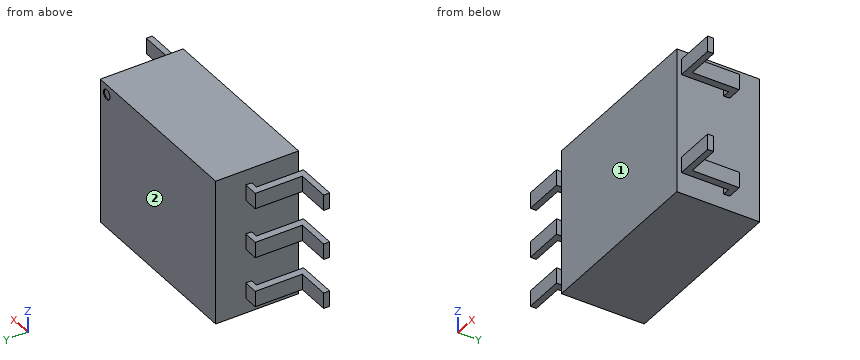
Autodesk Inventor part; units mm, degrees
ref_plane "YZ Plane" through (0, 0, 0) normal (1, 0, 0) x (0, 1, 0)
ref_plane "XZ Plane" through (0, 0, 0) normal (0, 1, 0) x (-1, 0, 0)
ref_plane "XY Plane" through (0, 0, 0) normal (0, 0, 1) x (1, 0, 0)
sketch "Sketch1" plane through (0, 0, 0) normal (0, 0, 1) x (1, 0, 0)
  line L0 (0, 0) -> (4.5491, 0)
  line L1 (4.5491, 0) -> (4.5491, 2.1006)
  line L2 (4.5491, 2.1006) -> (0, 2.1006)
  line L3 (0, 2.1006) -> (0, 0)
  dimension "d0" = 2.1006
  dimension "d1" = 4.5491
extrude "Extrusion1" add sketch "Sketch1" along normal blind 3.7008
sketch "Sketch2" plane through (4.5491, 0, 0) normal (1, 0, 0) x (0, 0, -1)
  line L0 (-3.3198, 1.3386) -> (-2.921, 1.3386)
  line L1 (-2.921, 1.3386) -> (-2.921, 1.1887)
  line L2 (-2.921, 1.1887) -> (-3.3198, 1.1887)
  line L3 (-3.3198, 1.1887) -> (-3.3198, 1.3386)
  line L4 (-0.7798, 1.3386) -> (-0.381, 1.3386)
  line L5 (-0.381, 1.3386) -> (-0.381, 1.1887)
  line L6 (-0.381, 1.1887) -> (-0.7798, 1.1887)
  line L7 (-0.7798, 1.1887) -> (-0.7798, 1.3386)
  line L8 (0, 0) -> (0, 2.1006)
  line L9 (0, 2.1006) -> (-3.7008, 2.1006)
  dimension "d4" = 0.3988
  dimension "d5" = 0.3988
  dimension "d6" = 0.1499
  dimension "d7" = 0.1499
  dimension "d8" = 2.1412
  dimension "d9" = 0
  dimension "d10" = 0.381
  dimension "d11" = 0.762
extrude "Extrusion2" add sketch "Sketch2" against normal blind 4.7727
extrude "Extrusion3" add sketch "Sketch2" along normal blind 0.2286
sketch "Sketch3" plane through (4.7777, 0, 0) normal (1, 0, 0) x (0, 0, -1)
  line L0 (-3.3198, 1.3386) -> (-2.921, 1.3386)
  line L1 (-2.921, 1.3386) -> (-2.921, 1.1887)
  line L2 (-2.921, 1.1887) -> (-3.3198, 1.1887)
  line L3 (-3.3198, 1.1887) -> (-3.3198, 1.3386)
  line L4 (-0.7798, 1.3386) -> (-0.381, 1.3386)
  line L5 (-0.381, 1.3386) -> (-0.381, 1.1887)
  line L6 (-0.381, 1.1887) -> (-0.7798, 1.1887)
  line L7 (-0.7798, 1.1887) -> (-0.7798, 1.3386)
  point P0 (0, 0)
extrude "Extrusion4" add sketch "Sketch3" along normal blind 0.1524
sketch "Sketch4" plane through (-0.2235, 0, 0) normal (-1, 0, 0) x (0, 0, 1)
  line L0 (2.921, 1.3386) -> (3.3198, 1.3386)
  line L1 (3.3198, 1.3386) -> (3.3198, 1.1887)
  line L2 (3.3198, 1.1887) -> (2.921, 1.1887)
  line L3 (2.921, 1.1887) -> (2.921, 1.3386)
  line L4 (0.381, 1.3386) -> (0.7798, 1.3386)
  line L5 (0.7798, 1.3386) -> (0.7798, 1.1887)
  line L6 (0.7798, 1.1887) -> (0.381, 1.1887)
  line L7 (0.381, 1.1887) -> (0.381, 1.3386)
  point P0 (0, 0)
extrude "Extrusion5" add sketch "Sketch4" along normal blind 0.1524
sketch "Sketch5" plane through (0, 1.1887, 2.921) normal (0, -1, 0) x (1, 0, 0)
  line L0 (0, -2.1412) -> (-0.3759, -2.1412)
  line L1 (-0.3759, -2.54) -> (-0.188, -2.54)
  line L2 (-0.188, -2.54) -> (-0.188, -2.1412)
  line L3 (-0.188, -2.1412) -> (-0.3759, -2.1412)
  line L4 (-0.3759, -2.1412) -> (-0.3759, -2.54)
  line L5 (0, 0.3988) -> (-0.3759, 0.3988)
  line L6 (-0.3759, 0) -> (-0.188, 0)
  line L7 (-0.188, 0) -> (-0.188, 0.3988)
  line L8 (-0.188, 0.3988) -> (-0.3759, 0.3988)
  line L9 (-0.3759, 0.3988) -> (-0.3759, 0)
  line L10 (4.5491, -2.1412) -> (4.9301, -2.1412)
  line L11 (4.9301, -2.54) -> (4.7396, -2.54)
  line L12 (4.7396, -2.54) -> (4.7396, -2.1412)
  line L13 (4.7396, -2.1412) -> (4.9301, -2.1412)
  line L14 (4.9301, -2.1412) -> (4.9301, -2.54)
  line L15 (4.5491, 0.3988) -> (4.9301, 0.3988)
  line L16 (4.9301, 0) -> (4.7396, 0)
  line L17 (4.7396, 0) -> (4.7396, 0.3988)
  line L18 (4.7396, 0.3988) -> (4.9301, 0.3988)
  line L19 (4.9301, 0.3988) -> (4.9301, 0)
  point P0 (0, -2.921)
extrude "Extrusion6" add sketch "Sketch5" along normal blind 1.1938
sketch "Sketch6" plane through (4.9301, 0, 0) normal (1, 0, 0) x (0, 0, -1)
  line L0 (-0.7798, 1.3386) -> (-0.7798, -0.0051)
  line L1 (-0.381, -0.0051) -> (-0.7798, -0.0051)
  line L2 (-0.7798, -0.0051) -> (-0.7798, 0.1473)
  line L3 (-0.7798, 0.1473) -> (-0.381, 0.1473)
  line L4 (-0.381, 0.1473) -> (-0.381, -0.0051)
  line L5 (-3.3198, 1.3386) -> (-3.3198, -0.0051)
  line L6 (-2.921, -0.0051) -> (-3.3198, -0.0051)
  line L7 (-3.3198, -0.0051) -> (-3.3198, 0.1473)
  line L8 (-3.3198, 0.1473) -> (-2.921, 0.1473)
  line L9 (-2.921, 0.1473) -> (-2.921, -0.0051)
  point P0 (0, 0)
  dimension "d22" = 0.1524
extrude "Extrusion7" add sketch "Sketch6" along normal blind 0.8433
sketch "Sketch7" plane through (-0.3759, 0, 0) normal (-1, 0, 0) x (0, 0, 1)
  line L0 (0.7798, -0.0051) -> (0.381, -0.0051)
  line L1 (0.381, -0.0051) -> (0.381, 0.1473)
  line L2 (0.381, 0.1473) -> (0.7798, 0.1473)
  line L3 (0.7798, 0.1473) -> (0.7798, -0.0051)
  line L4 (2.921, -0.0051) -> (3.3198, -0.0051)
  line L5 (3.3198, -0.0051) -> (3.3198, 0.1473)
  line L6 (3.3198, 0.1473) -> (2.921, 0.1473)
  line L7 (2.921, 0.1473) -> (2.921, -0.0051)
  point P0 (0, 0)
extrude "Extrusion8" add sketch "Sketch7" along normal blind 0.8433
sketch "Sketch8" plane through (0, 1.1887, 0.7798) normal (0, 0, 1) x (1, 0, 0)
  line L0 (0, 0) -> (0, 0.1499)
  line L1 (0, 0.1499) -> (-0.3759, 0.1499)
  line L2 (0, 0.1499) -> (-0.3759, 0.1499)
  line L3 (-0.3759, 0.1499) -> (-0.3759, -1.0414)
  line L4 (-0.3759, -1.0414) -> (-1.2192, -1.0414)
  line L5 (-1.2192, -1.0414) -> (-1.2192, -1.1938)
  line L6 (-0.188, -1.1938) -> (-1.2192, -1.1938)
  line L7 (-1.2192, -1.1938) -> (-0.188, -1.1938)
  line L8 (-0.188, -1.1938) -> (-0.188, 0)
  line L9 (-0.188, 0) -> (0, 0)
  line L10 (0, 0) -> (-0.188, 0)
  point P0 (0, -1.1887)
extrude "Extrusion9" add sketch "Sketch8" along normal blind 1.27
extrude "Extrusion10" cut sketch "Sketch8" along normal blind 0.8712
sketch "Sketch9" plane through (0, 2.1006, 0) normal (0, 1, 0) x (1, 0, 0)
  circle A0 centre (4.2951, -3.4468) radius 0.127
  line L0 (4.5491, 0) -> (4.5491, -3.7008)
  line L1 (4.5491, -3.7008) -> (0, -3.7008)
  point P0 (0, 0)
  dimension "d31" = 0.254
  dimension "d32" = 0.254
  dimension "d33" = 0.254
extrude "Extrusion11" cut sketch "Sketch9" against normal blind 0.0254
properties part number "sTLP152 Optocoupler"
Model file for the job. Use its own axes, mm. Face numbers are marked on the shaded views. Round coordinates to 2 decimals unless told otherwise and drop trailing zeros. Loops run counter-clockwise (first coordinate to the right, second up) from the corner with the lowest first, then second, coordinate; pieces in that order, holes last. Notation, with made-up numbers: (82, -31) - (131, -31) arc R20 ccw to (131, -3) - close; hole circle Ø1 at (-26.75, 66.25). An arc over 180 degrees is marked (long way). Write each question's results on one line, items separated by ' | '.
(1) Mould opens along X. For the marked faces 1 and 2 say: released by +X, released by -X, zero draft, split by the parting line, or undercut.
Answer below:
face 1: undercut | face 2: zero draft
(2) Wall check: L1, parallel to Z at x = -0.25, y = 1; L2, parallel to X at y = 0.9, z = 0.45; L3, parallel to Y at x = 0.5, z = 0.7. Give the ranges that are in metal, low to high.
Answer below:
L1: z = 0.38 to 0.78, 1.65 to 2.05, 2.92 to 3.32 | L2: x = -0.38 to -0.19, 0 to 4.55, 4.74 to 4.93 | L3: y = 0 to 2.1
(3) Saw through at C-C, the plane y = 1.9. List the corners of the cut face in (x, z).
Answer below:
outline: (0, 0) - (4.55, 0) - (4.55, 3.7) - (0, 3.7) - close
(4) Pin check, flat tip, straight feed: pin 1 (1.1 mm diameter, centred on y = 1.5, z = 3, fed in from +X). Stop position of the tip, or through.
Answer below:
pin 1: stops at x = 4.93
(5) Saw through at B-B, the plane z = 1.25. List the corners of the cut face in (x, y).
Answer below:
outline: (0, 0) - (4.55, 0) - (4.55, 2.1) - (0, 2.1) - close
(6) Saw through at A-A, the plane y = 1. List the corners of the cut face in (x, z), then the cut area to 3 significant figures.
Answer below:
outline: (-0.38, 0.38) - (-0.19, 0.38) - (-0.19, 0.78) - (-0.38, 0.78) - close; (-0.38, 1.65) - (-0.19, 1.65) - (-0.19, 2.05) - (-0.38, 2.05) - close; (-0.38, 2.92) - (-0.19, 2.92) - (-0.19, 3.32) - (-0.38, 3.32) - close; (0, 0) - (4.55, 0) - (4.55, 3.7) - (0, 3.7) - close; (4.74, 0.38) - (4.93, 0.38) - (4.93, 0.78) - (4.74, 0.78) - close; (4.74, 2.92) - (4.93, 2.92) - (4.93, 3.32) - (4.74, 3.32) - close | area: 17.2 mm^2
